```python
from build123d import *

# Parameters (mm, degrees)
SKETCH1_W           = 78
SKETCH1_H           = 78
SKETCH1_R           = 25.5
BOSS_EXTRUDE1_DEPTH = 110
CUT_EXTRUDE1_START  = -4
SKETCH2_R           = 29
CUT_EXTRUDE1_DEPTH  = 12
CUT_EXTRUDE2_START  = -16
SKETCH3_R           = 29
CUT_EXTRUDE2_DEPTH  = 12
THRUST_AX4565_R     = 35
THRUST_AX4565_R_2   = 25
CUT_EXTRUDE6_DEPTH  = 4
CUT_EXTRUDE7_START  = 4
SKETCH13_R          = 35
SKETCH13_R_2        = 25
CUT_EXTRUDE7_DEPTH  = 4
SKETCH8_R           = 2.5
CUT_EXTRUDE3_DEPTH  = 141.374499109


with BuildPart() as part:
    # Sketch1 → Boss-Extrude1 (new body)
    with BuildSketch(Plane.XY):
        Rectangle(SKETCH1_W, SKETCH1_H)
        Circle(SKETCH1_R, mode=Mode.SUBTRACT)
    extrude(amount=BOSS_EXTRUDE1_DEPTH)

    # Sketch2 → Cut-Extrude1 (cut)
    with BuildSketch(Plane(origin=(0, 0, 0), x_dir=(-1, 0, 0), z_dir=(0, 0, -1)).offset(CUT_EXTRUDE1_START)):
        Circle(SKETCH2_R)
    extrude(amount=-CUT_EXTRUDE1_DEPTH, mode=Mode.SUBTRACT)

    # Sketch3 → Cut-Extrude2 (cut)
    with BuildSketch(Plane.XY.offset(110).offset(CUT_EXTRUDE2_START)):
        with Locations(Location((0, 0, 0), (0, 0, 180))):
            Circle(SKETCH3_R)
    extrude(amount=CUT_EXTRUDE2_DEPTH, mode=Mode.SUBTRACT)

    # Thrust AX4565 → Cut-Extrude6 (cut)
    with BuildSketch(Plane.XY):
        Circle(THRUST_AX4565_R)
        Circle(THRUST_AX4565_R_2, mode=Mode.SUBTRACT)
    extrude(amount=CUT_EXTRUDE6_DEPTH, mode=Mode.SUBTRACT)

    # Sketch13 → Cut-Extrude7 (cut)
    with BuildSketch(Plane(origin=(0, 0, 110), x_dir=(-1, 0, 0), z_dir=(0, 0, -1)).offset(CUT_EXTRUDE7_START)):
        with Locations(Location((0, 0, 0), (0, 0, 180))):
            Circle(SKETCH13_R)
        Circle(SKETCH13_R_2, mode=Mode.SUBTRACT)
    extrude(amount=-CUT_EXTRUDE7_DEPTH, mode=Mode.SUBTRACT)

    # Sketch8 → Cut-Extrude3 (cut, through all)
    with BuildSketch(Plane(origin=(39, 0, 0), x_dir=(0, 0, -1), z_dir=(1, 0, 0))):
        with Locations(Location((-85, 32, 0), (0, 0, 90))):
            Circle(SKETCH8_R)
        with Locations(Location((-25, 32, 0), (0, 0, 90))):
            Circle(SKETCH8_R)
        with Locations(Location((-25, -32, 0), (0, 0, 90))):
            Circle(SKETCH8_R)
        with Locations(Location((-85, -32, 0), (0, 0, 90))):
            Circle(SKETCH8_R)
    extrude(amount=-CUT_EXTRUDE3_DEPTH, mode=Mode.SUBTRACT)


solid = part.part
```
Check sheet for the modelled part. Datum: model origin and axes. Units: mm. A direction names the side the tool comes from. Round coordinates to 2 decimals unless told otherwise and drop trailing zeros. Loops run counter-clockwise (first coordinate to the right, second up) from the corner with the lowest first, then second, coordinate; pieces in that order, holes last. Notation, with made-up numbers: (17, -9.75) - (22, -9.75) arc R15 cw to (22, 7.25) - close; hole circle Ø10 at (37.5, 88.25). An arc over 180 degrees is marked (long way). Answer as a JSON object with one key per item and string values. Group by question number.
Q1. Sectioned sample at B-B, the plane z = 25. Enter the section's corners in (x, y), plus the area to 3 significant figures.
Q2. Scan lines: line 1 along Z through (x, y) = (-2, -32); line 2 along Z through (x, y) = (16, -32); line 3 along Y through (x, z) = (-1, 33.5). Record each from-to range of solid material in increasing order. Write a range as [from, to].
Q3. Gauge pin test, flat ends, axial feed: P1, Ø2, axis at x = 28.5, y = 11, coming from the -Z side; P2, Ø21, axis at x = 4, y = 10.5, coming from the +Z side; P3, Ø17.5, axis at x = 11, y = -13, coming from the +Z side. Record the tip position at first contact, or that the pin passes through.
Q4. Sectioned sample at D-D, the plane z = 45.5. Enter the section's corners in (x, y), plus the area to 3 significant figures.
Q5. Mould release check, pull along Z, two halves, no side actions. Record for faces 4 (the face through (-13.1, -26.1, 106)), 5 (the face through (0.55, 31.67, 27.48)), 6 (the face through (-35.2, 0.5, 0)): released by +Z, released by -Z, zero draft, split by the parting line, or undercut.
Q6. Sectioned sample at A-A, the plane x = 0. Enter the section's corners in (y, z).
Q7. Sectioned sample at C-C, the plane y = 33. Enter the section's corners in (x, z), plus the area to 3 significant figures.
Q8. Set-up check for faces 1 (the face through (0, 26, 94)), 2 (the face through (0, -26, 16)), 3 (the face through (-1, 39, 54)): record each of +Z, -Z, +X, -X, +Y, -Y from which the full face is reachable in a straight line by a thin tool's end or side.
Solution:
{
 "1": {"outline": "(-39, -39) - (39, -39) - (39, -34.5) - (-39, -34.5) - close; (-39, -29.5) - (39, -29.5) - (39, 29.5) - (-39, 29.5) - close; (-39, 34.5) - (39, 34.5) - (39, 39) - (-39, 39) - close; hole circle Ø51 at (0, 0)", "area": "3,260 mm²"},
 "2": {"line 1": "z = [4, 22.5], [27.5, 82.5], [87.5, 106]", "line 2": "z = [0, 22.5], [27.5, 82.5], [87.5, 110]", "line 3": "y = [-39, -25.48], [25.48, 39]"},
 "3": {"P1": "stops at z = 4", "P2": "passes through", "P3": "stops at z = 94"},
 "4": {"outline": "(-39, -39) - (39, -39) - (39, 39) - (-39, 39) - close; hole circle Ø51 at (0, 0)", "area": "4,040 mm²"},
 "5": {"face 4": "released by +Z", "face 5": "undercut", "face 6": "released by -Z"},
 "6": {"outline": "(-39, 0) - (-35, 0) - (-35, 4) - (-29, 4) - (-29, 16) - (-25.5, 16) - (-25.5, 94) - (-29, 94) - (-29, 106) - (-35, 106) - (-35, 110) - (-39, 110) - close; (25.5, 16) - (29, 16) - (29, 4) - (35, 4) - (35, 0) - (39, 0) - (39, 110) - (35, 110) - (35, 106) - (29, 106) - (29, 94) - (25.5, 94) - close; hole circle Ø5 at (-32, 25); hole circle Ø5 at (-32, 85); hole circle Ø5 at (32, 25); hole circle Ø5 at (32, 85)"},
 "7": {"outline": "(-39, 0) - (-11.66, 0) - (-11.66, 4) - (11.66, 4) - (11.66, 0) - (39, 0) - (39, 22.71) - (-39, 22.71) - close; (-39, 27.29) - (39, 27.29) - (39, 82.71) - (-39, 82.71) - close; (-39, 87.29) - (39, 87.29) - (39, 110) - (11.66, 110) - (11.66, 106) - (-11.66, 106) - (-11.66, 110) - (-39, 110) - close", "area": "7,680 mm²"},
 "8": {"face 1": "+Z", "face 2": "-Z", "face 3": "+Z, -Z, +X, -X, +Y"}
}
